For this review, take the finished solid that the model builds, in its own axes (mm). A direction names the side the tool comes from. Give positions to 0.01 mm unless a question says otherwise; leave off trailing zeros. Write each loop counter-clockwise with the first axis right and the second up, starting at its lowest first coordinate (ties: lowest second). Pieces come first, ordered by that corner, then holes. Notation, with made-up numbers: M 10,11.5 L 21,11.5 A22 cw 21,28.5 Z; hole C -9.5,69.25 d2. An arc over 180 degrees is marked long. One line per item, written item: value. Start each with the question number.
Item 1: Consider section B-B, the plane y = -36.75. Write out the cut boundary in (x, z), and give its area (3 significant figures).
Item 2: To check wall thickness, follow probe 1 along Y at (x, z) = (-10.5, 7.5); probe 2 along Z at (x, y) = (10, -32.25); probe 3 along Z at (x, y) = (10, -34). State the ranges of each line that lie inside material, in increasing order.
Item 3: Tool access review of faces 4 (the face through (-13, -30, -1.535)), 5 (the face through (13, -30, -1.535)), 6 (the face through (3.396, -26, -17)), 7 (the face through (0, -26.94, 11)), 8 (the face through (0, -38.94, -2)): name each direction out of +Z, -Z, +X, -X, +Y, -Y from which nothing blocks a thin tool from reaching the whole face with its end or side.
Item 4: Consider section A-A, the plane y = -27.5. Write out the cut boundary in (x, z), and give its area (3 significant figures).
Item 5: Mouldability with a two-part tool opening along Y and no side actions: class faces 1 (the face through (0, -23.166, -17)), 2 (the face through (-0.26, -29.9, 10.46)), 3 (the face through (-3.204, -26, -17)) as released by +Y, released by -Y, zero draft, split by the parting line, or undercut.
Item 6: Clearance check with flat-ended pins moving along their axes: pin 1 Ø8 at (y, z) = (-36, 0) entering from +X; pin 2 Ø1.5 at (y, z) = (-26, -15) entering from -X; pin 3 Ø2 at (x, z) = (-0.5, -18) entering from -Y; pin 4 Ø6 at (y, z) = (-29, -10) entering from -X. State where each tip first meets the part, or that it passes through.
```python
from build123d import *

# Parameters (mm, degrees)
BOSS_EXTRUDE2_DEPTH = 60
BOSS_EXTRUDE3_DEPTH = 20
BOSS_EXTRUDE5_START = -40
BOSS_EXTRUDE5_DEPTH = 20
FILLET2_START       = -43.0000001
FILLET2_OUTLINE_R   = 50
FILLET2_DEPTH       = 3.0000001
FILLET2_START_2     = -20
FILLET2_2_OUTLINE_R = 50
FILLET2_2_DEPTH     = 3.0000001
FILLET2_START_3     = -40
FILLET2_3_DEPTH     = 20
FILLET2_START_4     = -56.0000001
FILLET2_5_DEPTH     = 42.000000197
SKETCH2_W           = 22
SKETCH2_H           = 16
BOSS_EXTRUDE6_DEPTH = 5
SKETCH2_2_W         = 22
SKETCH2_2_H         = 16
BOSS_EXTRUDE7_DEPTH = 7
SCALE6_SCALE        = 0.3


with BuildPart() as part:
    # Sketch1 → Boss-Extrude2 (new body)
    with BuildSketch(Plane(origin=(0, 0, 0), x_dir=(1, 0, 0), z_dir=(0, 1, 0))):
        with BuildLine():
            ThreePointArc((-40, 0), (0, -40), (40, 0))
            Line((40, 0), (50, 0))
            ThreePointArc((50, 0), (0, 50), (-50, 0))
            Line((-50, 0), (-40, 0))
        make_face()
    extrude(amount=-BOSS_EXTRUDE2_DEPTH)

    # Sketch1<4> → Boss-Extrude3 (add)
    with BuildSketch(Plane(origin=(0, 0, 0), x_dir=(1, 0, 0), z_dir=(0, 1, 0))):
        with BuildLine():
            ThreePointArc((-40, 0), (0, -40), (40, 0))
            Line((40, 0), (50, 0))
            ThreePointArc((50, 0), (0, 50), (-50, 0))
            Line((-50, 0), (-40, 0))
        make_face()
        with BuildLine():
            Line((50, 0), (40, 0))
            ThreePointArc((40, 0), (0, -40), (-40, 0))
            Line((-40, 0), (-50, 0))
            ThreePointArc((-50, 0), (0, -50), (50, 0))
        make_face()
    extrude(amount=-BOSS_EXTRUDE3_DEPTH)

    # Sketch1<6> → Boss-Extrude5 (add)
    with BuildSketch(Plane(origin=(0, 0, 0), x_dir=(1, 0, 0), z_dir=(0, 1, 0)).offset(BOSS_EXTRUDE5_START)):
        with BuildLine():
            ThreePointArc((-40, 0), (0, -40), (40, 0))
            Line((40, 0), (50, 0))
            ThreePointArc((50, 0), (0, 50), (-50, 0))
            Line((-50, 0), (-40, 0))
        make_face()
        with BuildLine():
            Line((50, 0), (40, 0))
            ThreePointArc((40, 0), (0, -40), (-40, 0))
            Line((-40, 0), (-50, 0))
            ThreePointArc((-50, 0), (0, -50), (50, 0))
        make_face()
    extrude(amount=-BOSS_EXTRUDE5_DEPTH)

    # Fillet1: read off the stored shape, not the designer's step
    # Fillet1 outline → Fillet1 (revolve, cut)
    with BuildSketch(Plane.XY):
        with BuildLine():
            ThreePointArc((46, 0), (48.828427125, -1.171572875), (50, -4))
            Line((50, -4), (50, 0))
            Line((50, 0), (46, 0))
        make_face()
        with BuildLine():
            Line((50, -60), (50, -56))
            ThreePointArc((50, -56), (48.828427125, -58.828427125), (46, -60))
            Line((46, -60), (50, -60))
        make_face()
    revolve(axis=Axis((0, 0, 0), (0, 1, 0)), mode=Mode.SUBTRACT)

    # Fillet2: read off the stored shape, not the designer's step
    # Fillet2 outline → Fillet2 (cut)
    with BuildSketch(Plane(origin=(0, 0, 0), x_dir=(1, 0, 0), z_dir=(0, 1, 0)).offset(FILLET2_START)):
        Circle(FILLET2_OUTLINE_R)
    extrude(amount=FILLET2_DEPTH, mode=Mode.SUBTRACT)

    # Fillet2 2 outline → Fillet2 2 (cut)
    with BuildSketch(Plane(origin=(0, 0, 0), x_dir=(1, 0, 0), z_dir=(0, 1, 0)).offset(FILLET2_START_2)):
        Circle(FILLET2_2_OUTLINE_R)
    extrude(amount=FILLET2_2_DEPTH, mode=Mode.SUBTRACT)

    # Fillet2 3 outline → Fillet2 3 (cut)
    with BuildSketch(Plane(origin=(0, 0, 0), x_dir=(1, 0, 0), z_dir=(0, 1, 0)).offset(FILLET2_START_3)):
        with BuildLine():
            ThreePointArc((49.898039998, 3.191489362), (49.092132471, 0.947497635), (46.904157598, 0))
            Line((46.904157598, 0), (50, 0))
            ThreePointArc((50, 0), (49.974503499, 1.596558814), (49.898039998, 3.191489362))
        make_face()
        with BuildLine():
            ThreePointArc((-46.904157598, 0), (-49.092132471, 0.947497635), (-49.898039998, 3.191489362))
            ThreePointArc((-49.898039998, 3.191489362), (-49.974503499, 1.596558814), (-50, 0))
            Line((-50, 0), (-46.904157598, 0))
        make_face()
    extrude(amount=FILLET2_3_DEPTH, mode=Mode.SUBTRACT)

    # Fillet2 4 outline → Fillet2 4 (revolve)
    with BuildSketch(Plane.XY):
        with BuildLine():
            Line((0, -17), (0, -20))
            Line((0, -20), (47, -20))
            ThreePointArc((47, -20), (49.121320344, -19.121320344), (50, -17))
            Line((50, -17), (0, -17))
        make_face()
        with BuildLine():
            Line((47, -40), (0, -40))
            Line((0, -40), (0, -43))
            Line((0, -43), (50, -43))
            ThreePointArc((50, -43), (49.121320344, -40.878679656), (47, -40))
        make_face()
    revolve(axis=Axis((0, 0, 0), (0, 1, 0)))

    # Fillet2 5 outline → Fillet2 5 (add)
    with BuildSketch(Plane(origin=(0, 0, 0), x_dir=(1, 0, 0), z_dir=(0, 1, 0)).offset(FILLET2_START_4)):
        with BuildLine():
            ThreePointArc((46.904157598, 0), (49.092132471, 0.947497635), (49.898039998, 3.191489362))
            ThreePointArc((49.898039998, 3.191489362), (0, 50), (-49.898039998, 3.191489362))
            ThreePointArc((-49.898039998, 3.191489362), (-49.092132471, 0.947497635), (-46.904157598, 0))
            Line((-46.904157598, 0), (46.904157598, 0))
        make_face()
    extrude(amount=FILLET2_5_DEPTH)

    # Sketch2 → Boss-Extrude6 (add)
    with BuildSketch(Plane.XY.offset(-50)):
        with Locations((0.314864649, -15.421130919)):
            Rectangle(SKETCH2_W, SKETCH2_H)
    extrude(amount=BOSS_EXTRUDE6_DEPTH)

    # Sketch2<2> → Boss-Extrude7 (add)
    with BuildSketch(Plane.XY.offset(-50)):
        with Locations((0.314864649, -15.421130919)):
            Rectangle(SKETCH2_2_W, SKETCH2_2_H)
    extrude(amount=-BOSS_EXTRUDE7_DEPTH)


with BuildPart() as part_1:
    # Scale6: scaled about (0.002059133, -29.914145752, -2.193081509)
    add(part.part.scale(SCALE6_SCALE).moved(Location((0.001441393, -20.939902026, -1.535157056))))


solid = part_1.part
```
Model answer:
1. outline: C 0,-1.54 d30
1. area: 707 mm2
2. probe 1: y = -38.94 to -32.94, -26.94 to -20.94
2. probe 2: z = -12.72 to 5.1
2. probe 3: z = -12.72 to 9.65
3. face 4: +Z, -X
3. face 5: +Z, +X
3. face 6: -Z, +X, +Y, -Y
3. face 7: +Z
3. face 8: +Z, -Z, +X, -X, -Y
4. outline: M -14.97,-2.49 A15 ccw -3.2,-16.19 L -3.2,-18.64 L 3.4,-18.64 L 3.4,-16.15 A15 ccw 14.97,-2.49 A0.9 ccw 14.07,-1.54 L 12,-1.54 A12 ccw -12,-1.54 L -14.07,-1.54 A0.9 ccw Z
4. area: 594 mm2
5. face 1: released by +Y
5. face 2: undercut
5. face 3: zero draft
6. pin 1: stops at x = 15
6. pin 2: stops at x = -7.96
6. pin 3: stops at y = -27.97
6. pin 4: stops at x = -13.97
